For this review, take the finished solid that the model builds, in its own axes (mm). A direction names the side the tool comes from. Coordinates: 2 decimals unless noted, no trailing zeros. Loops run counter-clockwise (first coordinate to the right, second up) from the corner with the lowest first, then second, coordinate; pieces in that order, holes last.
```python
from build123d import *

# Parameters (mm, degrees)
SKETCH1_R           = 3.1
BOSS_EXTRUDE1_DEPTH = 8


with BuildPart() as part:
    # Sketch1 → Boss-Extrude1 (new body)
    with BuildSketch(Plane.XY):
        Polygon((-35, 0), (-35, 37), (-31.5, 37), (-31.5, 34), (-27, 34), (-27, 31), (-22.5, 31), (-22.5, 28), (-18, 28), (-18, 25), (-13.5, 25), (-13.5, 22), (-9, 22), (-9, 19), (-4.5, 19), (-4.5, 16), (0, 16), (0, 0), align=None)
        with Locations((-24, 12)):
            Circle(SKETCH1_R, mode=Mode.SUBTRACT)
    boss_extrude1 = extrude(amount=BOSS_EXTRUDE1_DEPTH)

    # Mirror1: Boss-Extrude1 across plane
    add(boss_extrude1.mirror(Plane(origin=(0, 0, 0), x_dir=(0, 0, 1), z_dir=(1, 0, 0))))


solid = part.part
```
Q1. Machinability: for faces 1 (the face through (0, 0, 4)), 2 (the face through (-18, 27, 4)), which of the approach directions +Z, -Z, +X, -X, +Y, -Y give a long, thin tool a straight path to every point of the face, cutting with its end or side? Answer none if there is none.
Q2. For pin 1 Ø3.5 at (x, z) = (-19.5, 5) entering from +Y; pin 2 Ø2 at (x, z) = (5.5, 5.5) entering from +Y; pin 3 Ø3.5 at (x, z) = (-12, 4) entering from +Y; pin 4 Ø4 at (x, y) = (7, 24) entering from -Z, all flat-tipped, find the tip position at first contact; note any pin that passes through.
Q3. Consider section A-A (y = 12). State the section outline as (x, z) points, then the cut area to 3 significant figures.
Q4. Consider section C-C (z = 4.5). Count the separate pieces of the cut face and the enclosed holes in it, then the cut area to 3 significant figures.
Q5. Consider section B-B (x = 24). State the section outline as (y, z) points, then the cut area to 3 significant figures.
Q6. Wall thickness on probe 1 along Y at (x, z) = (-24, 5.75); probe 2 along X at (y, z) = (14.5, 7.5); probe 3 along X at (y, z) = (11, 4.25): over which ranges is each line inside the solid? List them lowest first.
Q7. Consider section D-D (y = 29). State the section outline as (x, z) points.
Q8. The part is to be moulded in two halves that separate along X. For faces 3 (the face through (-20, 28, 4)), 4 (the face through (0, 15, 8)), 5 (the face through (29, 34, 4)), say which applies: +X half, -X half, draft (parallel to the pull), parting line (faces both ways), or undercut.
Model answer:
1. face 1: +Z, -Z, +X, -X, -Y
1. face 2: +Z, -Z, +Y
2. pin 1: stops at y = 28
2. pin 2: stops at y = 19
2. pin 3: stops at y = 25
2. pin 4: passes through
3. outline: (-35, 0) - (-27.1, 0) - (-27.1, 8) - (-35, 8) - close; (-20.9, 0) - (20.9, 0) - (20.9, 8) - (-20.9, 8) - close; (27.1, 0) - (35, 0) - (35, 8) - (27.1, 8) - close
3. area: 461 mm2
4. separate pieces: 1
4. enclosed holes: 2
4. area: 1,770 mm2
5. outline: (0, 0) - (8.9, 0) - (8.9, 8) - (0, 8) - close; (15.1, 0) - (31, 0) - (31, 8) - (15.1, 8) - close
5. area: 198 mm2
6. probe 1: y = 0 to 8.9, 15.1 to 31
6. probe 2: x = -35 to -25.83, -22.17 to 22.17, 25.83 to 35
6. probe 3: x = -35 to -26.93, -21.07 to 21.07, 26.93 to 35
7. outline: (-35, 0) - (-22.5, 0) - (-22.5, 8) - (-35, 8) - close; (22.5, 0) - (35, 0) - (35, 8) - (22.5, 8) - close
8. face 3: undercut
8. face 4: draft
8. face 5: undercut
